```python
from build123d import *

# Parameters (mm, degrees)
SKETCH1_W           = 260
SKETCH1_H           = 115
SKETCH1_W_2         = 78.493115051
SKETCH1_H_2         = 64
BOSS_EXTRUDE1_DEPTH = 10


with BuildPart() as part:
    # Sketch1 → Boss-Extrude1 (new body)
    with BuildSketch(Plane(origin=(0, 0, 0), x_dir=(1, 0, 0), z_dir=(0, 1, 0))):
        with Locations((-130, 57.5)):
            Rectangle(SKETCH1_W, SKETCH1_H)
        with BuildLine():
            ThreePointArc((-247.5, 89.5), (-251.035533906, 88.035533906), (-252.5, 84.5))
            Line((-252.5, 84.5), (-252.5, 30.5))
            ThreePointArc((-252.5, 30.5), (-251.035533906, 26.964466094), (-247.5, 25.5))
            Line((-247.5, 25.5), (-175.5, 25.5))
            ThreePointArc((-175.5, 25.5), (-171.964466094, 26.964466094), (-170.5, 30.5))
            Line((-170.5, 30.5), (-170.5, 84.5))
            ThreePointArc((-170.5, 84.5), (-171.964466094, 88.035533906), (-175.5, 89.5))
            Line((-175.5, 89.5), (-247.5, 89.5))
        make_face(mode=Mode.SUBTRACT)
        with Locations((-46.746557526, 57.5)):
            Rectangle(SKETCH1_W_2, SKETCH1_H_2, mode=Mode.SUBTRACT)
    extrude(amount=BOSS_EXTRUDE1_DEPTH)


solid = part.part
```
The listing builds one solid part. Answer for the finished solid, in the listing's coordinates (mm). A direction names the side the tool comes from. Coordinates: 2 decimals unless noted, no trailing zeros. Loops run counter-clockwise (first coordinate to the right, second up) from the corner with the lowest first, then second, coordinate; pieces in that order, holes last. Notation, with made-up numbers: (-22, 21) -> (22, 21) arc R10 cw to (22, 32) -> close; hole circle Ø5 at (32.25, 59.25). An arc over 180 degrees is marked (long way). Return JSON: item names as keys, results as strings. Group by question number.
(1) A cutting plane is placed at A-A on x = -78. Write down the section's boundary in (y, z), and give its area (3 significant figures).
(2) Which of the six approach directions +Z, -Z, +X, -X, +Y, -Y give full straight-line access (tool end or side, diameter ignored) to faces 1 (the flat face through (-7.5, 5, -57)), 2 (the flat face through (-132, 10, -58))?
(3) A cutting plane is placed at C-C on y = 6.75. Write down the section's boundary in (x, z), and give its area (3 significant figures).
(4) Find the intervals of material crossed by probe 1 along X at (y, z) = (8.5, -62); probe 2 along Z at (x, y) = (-36, 3.5); probe 3 along Z at (x, y) = (-171.5, 8.75), in increasing order. Write a range as from..to.
(5) A cutting plane is placed at B-B on z = -57.5. Write down the section's boundary in (x, y).
(6) Determine the mould class of faces 3 (the flat face through (-212, 5, -25.5)), 4 (the flat face through (-132, 5, 0)), 5 (the flat face through (-132, 0, -58)) for opening direction Z: released by +Z, released by -Z, zero draft, split by the parting line, or undercut.
The answers:
{
 "1": {"outline": "(0, -115) -> (10, -115) -> (10, -89.5) -> (0, -89.5) -> close; (0, -25.5) -> (10, -25.5) -> (10, 0) -> (0, 0) -> close", "area": "510 mm^2"},
 "2": {"face 1": "+Y, -Y", "face 2": "+Z, -Z, +X, -X, +Y"},
 "3": {"outline": "(-260, -115) -> (0, -115) -> (0, 0) -> (-260, 0) -> close; hole (-252.5, -84.5) arc R5 ccw to (-247.5, -89.5) -> (-175.5, -89.5) arc R5 ccw to (-170.5, -84.5) -> (-170.5, -30.5) arc R5 ccw to (-175.5, -25.5) -> (-247.5, -25.5) arc R5 ccw to (-252.5, -30.5) -> close; hole (-85.99, -89.5) -> (-7.5, -89.5) -> (-7.5, -25.5) -> (-85.99, -25.5) -> close", "area": "19,600 mm^2"},
 "4": {"probe 1": "x = -260..-252.5, -170.5..-85.99, -7.5..0", "probe 2": "z = -115..-89.5, -25.5..0", "probe 3": "z = -115..-87.5, -27.5..0"},
 "5": {"outline": "(-260, 0) -> (-252.5, 0) -> (-252.5, 10) -> (-260, 10) -> close; (-170.5, 0) -> (-85.99, 0) -> (-85.99, 10) -> (-170.5, 10) -> close; (-7.5, 0) -> (0, 0) -> (0, 10) -> (-7.5, 10) -> close"},
 "6": {"face 3": "undercut", "face 4": "released by +Z", "face 5": "zero draft"}
}
